Verification items for the finished model (mm, model axes). Face numbers are marked on the shaded views. A direction names the side the tool comes from. Give positions to 0.01 mm unless a question says otherwise; leave off trailing zeros. Write each loop counter-clockwise with the first axis right and the second up, starting at its lowest first coordinate (ties: lowest second). Pieces come first, ordered by that corner, then holes. Notation, with made-up numbers: (65.5, 34) -> (99.5, 34) arc R14 ccw to (99.5, 54) -> close; hole circle Ø3 at (41.5, 75). An arc over 180 degrees is marked (long way). Write item = value, one per line.
from build123d import *

# Parameters (mm, degrees)
F0_R     = 35
F1_DEPTH = 4
F2_R     = 2.75
F3_DEPTH = 4
F4_R     = 26
F5_DEPTH = 3
F6_R     = 21
F7_DEPTH = 4
F8_SIZE  = 1


with BuildPart() as f1:
    # F0 (on Front) → F1 (new body)
    with BuildSketch(Plane.XZ):
        Circle(F0_R)
    extrude(amount=F1_DEPTH)

    # F2 (on face) → F3 (cut, through all)
    with BuildSketch(Plane.XZ.offset(4)):
        with Locations((30, 0)):
            Circle(F2_R)
        with Locations((0, 30)):
            Circle(F2_R)
        with Locations((-30, 0)):
            Circle(F2_R)
        with Locations((0, -30)):
            Circle(F2_R)
    extrude(amount=-F3_DEPTH, mode=Mode.SUBTRACT)

    # F4 (on face) → F5 (join)
    with BuildSketch(Plane.XZ.offset(4)):
        Circle(F4_R)
    extrude(amount=F5_DEPTH)

    # F6 (on face) → F7 (cut)
    with BuildSketch(Plane.XZ.offset(7)):
        Circle(F6_R)
    extrude(amount=-F7_DEPTH, mode=Mode.SUBTRACT)

    # F8
    f8_edges = [f1.edges().sort_by_distance(p)[0] for p in [
        (-26, -7, 0),
    ]]
    chamfer(f8_edges, length=F8_SIZE)


solid = f1.part
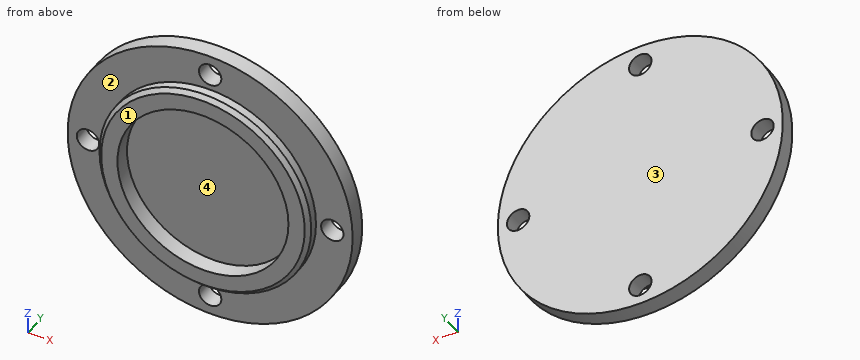
Item 1: Sectioned sample at C-C on x = 30. Record the cut outline in (y, z).
Response values:
outline = (-4, -18.03) -> (0, -18.03) -> (0, -2.75) -> (-4, -2.75) -> close; (-4, 2.75) -> (0, 2.75) -> (0, 18.03) -> (-4, 18.03) -> close
Item 2: Go/stop test with flat-tipped pins: P1, Ø9, axis at x = 0, z = -30, coming from the +Y side; P2, Ø1.5, axis at x = 2.5, y = -5.5, coming from the +Z side; P3, Ø1.5, axis at x = -24, y = -6, coming from the -Z side. Record where each tip stops, or that it passes through.
Response values:
P1 = 0
P2 = 25.94
P3 = -11.64
Item 3: Sectioned sample at A-A on x = 0. Record the cut outline in (y, z).
Response values:
outline = (-7, -25) -> (-6, -26) -> (-4, -26) -> (-4, -27.25) -> (0, -27.25) -> (0, 27.25) -> (-4, 27.25) -> (-4, 26) -> (-6, 26) -> (-7, 25) -> (-7, 21) -> (-3, 21) -> (-3, -21) -> (-7, -21) -> close; (-4, -35) -> (0, -35) -> (0, -32.75) -> (-4, -32.75) -> close; (-4, 32.75) -> (0, 32.75) -> (0, 35) -> (-4, 35) -> close
Item 4: Mould release check, pull along X, two halves, no side actions. Record for the marked faces 3 and 4: +X half, -X half, draft (parallel to the pull), parting line (faces both ways), or undercut.
Response values:
face_3 = draft
face_4 = undercut
Item 5: Sectioned sample at B-B on z = 0. Record the cut outline in (x, y).
Response values:
outline = (-35, -4) -> (-32.75, -4) -> (-32.75, 0) -> (-35, 0) -> close; (-27.25, -4) -> (-26, -4) -> (-26, -6) -> (-25, -7) -> (-21, -7) -> (-21, -3) -> (21, -3) -> (21, -7) -> (25, -7) -> (26, -6) -> (26, -4) -> (27.25, -4) -> (27.25, 0) -> (-27.25, 0) -> close; (32.75, -4) -> (35, -4) -> (35, 0) -> (32.75, 0) -> close
Item 6: Set-up check for the marked faces 1 and 2: record each of +Z, -Z, +X, -X, +Y, -Y from which the full face is reachable in a straight line by a thin tool's end or side.
Response values:
face_1 = +Z, -Z, +X, -X, -Y
face_2 = -Y
Item 7: Material ranges on line 1 (Z direction, x = 0, y = -1.95); line 2 (Y direction, x = -28.5, z = 16); line 3 (Y direction, x = 1, z = 11.5), recorded low to high.
Response values:
line_1 = -35 to -32.75, -27.25 to 27.25, 32.75 to 35
line_2 = -4 to 0
line_3 = -3 to 0
Item 8: Sectioned sample at D-D on z = 30. Record the cut outline in (x, y), then the cut area to 3 significant figures.
Response values:
outline = (-18.03, -4) -> (-2.75, -4) -> (-2.75, 0) -> (-18.03, 0) -> close; (2.75, -4) -> (18.03, -4) -> (18.03, 0) -> (2.75, 0) -> close
area = 122 mm^2
